Autodesk Inventor part; units mm, degrees
ref_plane "YZ Plane" through (0, 0, 0) normal (1, 0, 0) x (0, 1, 0)
ref_plane "XZ Plane" through (0, 0, 0) normal (0, 1, 0) x (-1, 0, 0)
ref_plane "XY Plane" through (0, 0, 0) normal (0, 0, 1) x (1, 0, 0)
sketch "スケッチ1" plane through (0, 0, 0) normal (0, 0, 1) x (1, 0, 0)
  circle A0 centre (0, 0) radius 1.5
  dimension "d0" = 3
extrude "押し出し1" add sketch "スケッチ1" along normal blind 20
sketch "スケッチ2" plane through (0, 0, 0) normal (0, 0, -1) x (-1, 0, 0)
  circle A0 centre (0, 0) radius 2.75
  dimension "d3" = 5.5
extrude "押し出し2" add sketch "スケッチ2" along normal blind 2
fillet "フィレット1" radius 2 1 edges at (2.75, 0, -2)
thread "ねじ1"
properties part number "ネジ鍋m3,20" material "鋼、高強度、低合金"
Model file for the job. Use its own axes, mm. A direction names the side the tool comes from. Round coordinates to 2 decimals unless told otherwise and drop trailing zeros. Write each loop counter-clockwise with the first axis right and the second up, starting at its lowest first coordinate (ties: lowest second). Pieces come first, ordered by that corner, then holes. Notation, with made-up numbers: (20.5, 8) - (50.5, 8) arc R21 ccw to (50.5, 21) - close; hole circle Ø11 at (57.5, 36.5). An arc over 180 degrees is marked (long way). Use CSV: the item, a comma, the result in double quotes. Start each with the question number.
Item 1: Tool access for faces 1 (the face through (0, 0, 20)), 2 (the face through (-1.2, -1.2, 0)): list every direction of +Z, -Z, +X, -X, +Y, -Y with a clear straight run to the whole face (end or side of a thin tool).
Item 2: Drill centre lines: L1, parallel to Y at x = 0.1, z = 8; L2, parallel to Z at x = 0.15, y = -2.4. Where is each one in solid material? Low to high. Write a range as [from, to].
Item 3: Pin check, flat tip, straight feed: P1, Ø2, axis at x = 1, z = 7.5, coming from the -Y side. Stop position of the tip, or through.
Item 4: Band-saw the part on A-A (z = 11.75). Write the cut outline in (x, y).
Checked values:
1,face 1,"+Z, +X, -X, +Y, -Y"
1,face 2,"+Z"
2,L1,"y = [-1.5, 1.5]"
2,L2,"z = [-1.12, 0]"
3,P1,"stops at y = -1.5"
4,outline,"circle Ø3 at (0, 0)"
